The listing builds one solid part. Answer for the finished solid, in the listing's coordinates (mm). Round coordinates to 2 decimals unless told otherwise and drop trailing zeros. Order: outer loops, then holes, each group sorted by start corner. A loop starts at its lowest first (then second) coordinate and runs counter-clockwise, first axis right, second up. Notation, with made-up numbers: M 43,37.25 L 47,37.25 A24 ccw 47,76.25 Z; hole C 58,-9.5 d7. An arc over 180 degrees is marked long. Write item = value, one per line. Start each with the question number.
(1) A cutting plane is placed at D-D, the plane x = 11.5. Determine the outline of the cut face in (y, z).
(2) Each of these flat-tipped pins is pushed along its axis until it touches: pin 1 (1.7 mm diameter, centred on x = 0, y = 0.5, fed in from +Z); pin 2 (5 mm diameter, centred on x = 5.5, z = 31.5, fed in from +Y); pin 3 (0.8 mm diameter, centred on y = -2.5, z = 21, fed in from -X); pin 4 (4 mm diameter, centred on x = 8, z = 33.5, fed in from +Y). Where does it stop, or does it pass through?
(3) A cutting plane is placed at C-C, the plane y = -1.05. Determine the outline of the cut face in (x, z).
(4) A cutting plane is placed at B-B, the plane x = 8. Determine the outline of the cut face in (y, z), and give its area (3 significant figures).
(5) Straight lines are drawn through the part: probe 1 along Z at (x, y) = (8, -2.6); probe 2 along Z at (x, y) = (7.25, -2); probe 3 along Z at (x, y) = (1, -1.6). For each, find the intervals that lie inside material, in ascending order. Write a range as from..to.
(6) A cutting plane is placed at A-A, the plane z = 33.5. Determine the outline of the cut face in (x, y).
from build123d import *

# Parameters (mm, degrees)
ESQUISSE1_R                  = 1.75
BOSS_EXTRU_1_DEPTH           = 40
ENL_V_MAT_EXTRU_3_DEPTH      = 20
ENL_V_MAT_EXTRU_3_DEPTH_BACK = 20
ESQUISSE2_W                  = 17.8
ESQUISSE2_H                  = 8
D_GAGEMENT_M31_D             = 3
D_GAGEMENT_M31_DEPTH         = 10
D_GAGEMENT_M31_CSINK_D       = 4.4
D_GAGEMENT_M31_CSINK_ANGLE   = 90
D_GAGEMENT_M31_TIP           = 0.901290929


with BuildPart() as part:
    # Esquisse1 → Boss.-Extru.1 (new body)
    with BuildSketch(Plane.XY):
        with BuildLine():
            Line((12.5, -1.75), (2.121320344, -1.75))
            ThreePointArc((2.121320344, -1.75), (-1.17260394, 2.487468593), (0, -2.75))
            Line((0, -2.75), (12.5, -2.75))
            Line((12.5, -2.75), (12.5, -1.75))
        make_face()
        Circle(ESQUISSE1_R, mode=Mode.SUBTRACT)
    extrude(amount=BOSS_EXTRU_1_DEPTH)

    # Esquisse2 → Enlèv. mat.-Extru.3 (cut, two sides: drawn at the far end of the back side and taken through both)
    with BuildSketch(Plane(origin=(0, -1.75, 0), x_dir=(1, 0, 0), z_dir=(0, 1, 0)).offset(-ENL_V_MAT_EXTRU_3_DEPTH_BACK)):
        with Locations((-5.3, -20)):
            Rectangle(ESQUISSE2_W, ESQUISSE2_H)
        with Locations((-5.3, -36)):
            Rectangle(ESQUISSE2_W, ESQUISSE2_H)
        with Locations((-5.3, -4)):
            Rectangle(ESQUISSE2_W, ESQUISSE2_H)
    extrude(amount=ENL_V_MAT_EXTRU_3_DEPTH + ENL_V_MAT_EXTRU_3_DEPTH_BACK, mode=Mode.SUBTRACT)

    # Dégagement M31
    with Locations(Plane(origin=(0, -1.75, 0), x_dir=(1, 0, 0), z_dir=(0, 1, 0))):
        with Locations((8, -33.5), (8, -6.5)):
            CounterSinkHole(D_GAGEMENT_M31_D / 2, D_GAGEMENT_M31_CSINK_D / 2, depth=D_GAGEMENT_M31_DEPTH, counter_sink_angle=D_GAGEMENT_M31_CSINK_ANGLE)
            with Locations((0, 0, -(D_GAGEMENT_M31_DEPTH + D_GAGEMENT_M31_TIP / 2))):  # 118° drill point
                Cone(0, D_GAGEMENT_M31_D / 2, D_GAGEMENT_M31_TIP, mode=Mode.SUBTRACT)


solid = part.part
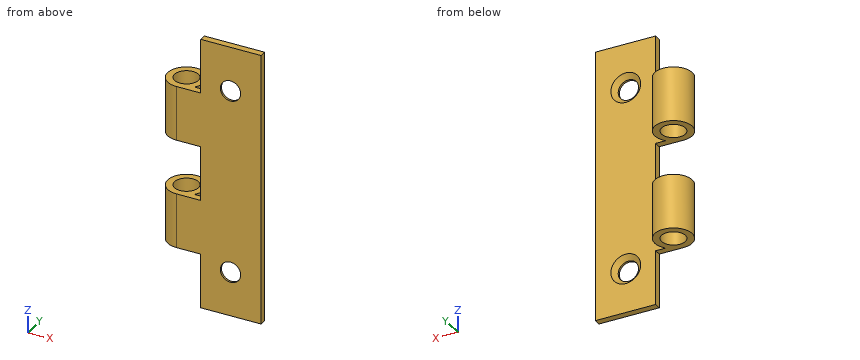
Reported:
q1.outline = M -2.75,0 L -1.75,0 L -1.75,40 L -2.75,40 Z
q2.pin_1 = through
q2.pin_2 = -1.75
q2.pin_3 = 3.6
q2.pin_4 = -1.95
q3.outline = M -2.54,8 L -1.4,8 L -1.4,16 L -2.54,16 Z; M -2.54,24 L -1.4,24 L -1.4,32 L -2.54,32 Z; M 1.4,8 L 2.54,8 L 2.54,16 L 1.4,16 Z; M 1.4,24 L 2.54,24 L 2.54,32 L 1.4,32 Z
q4.outline = M -2.75,0 L -1.75,0 L -1.75,4.3 L -2.45,5 L -2.75,5 Z; M -2.75,8 L -2.45,8 L -1.75,8.7 L -1.75,31.3 L -2.45,32 L -2.75,32 Z; M -2.75,35 L -2.45,35 L -1.75,35.7 L -1.75,40 L -2.75,40 Z
q4.area = 33.0 mm²
q5.probe_1 = 0..5, 8..32, 35..40
q5.probe_2 = 0..4.7, 8.3..31.7, 35.3..40
q5.probe_3 = 8..16, 24..32
q6.outline = M 3.6,-2.75 L 6.5,-2.75 L 6.5,-2.45 L 5.8,-1.75 L 3.6,-1.75 Z; M 9.5,-2.75 L 12.5,-2.75 L 12.5,-1.75 L 10.2,-1.75 L 9.5,-2.45 Z
